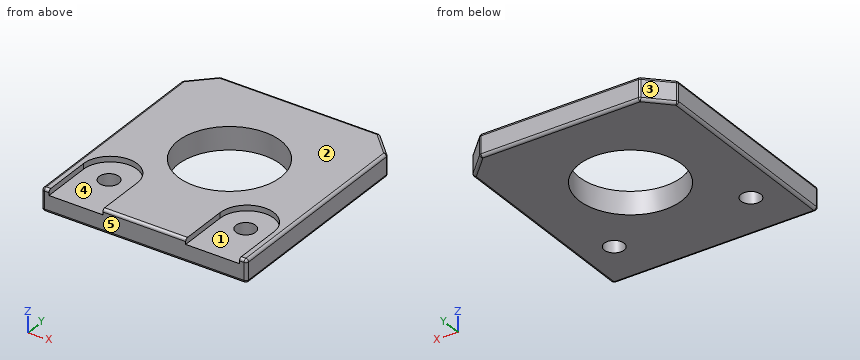
```python
from build123d import *

# Parameters (mm, degrees)
SKETCH2_W            = 57.15
SKETCH2_H            = 6.35
BOSS_EXTRUDE1_DEPTH  = 63.5
SKETCH3_R            = 14.2875
CUT_EXTRUDE1_DEPTH   = 70.922121857
CHAMFER1_SIZE        = 6.35
M5_CLEARANCE_HOLE1_D = 5.5
FILLET1_R            = 0.762
CUT_EXTRUDE4_DEPTH   = 1.524


with BuildPart() as part:
    # Sketch2 → Boss-Extrude1 (new body)
    with BuildSketch(Plane(origin=(0, 0, 0), x_dir=(1, 0, 0), z_dir=(0, 1, 0))):
        Rectangle(SKETCH2_W, SKETCH2_H)
    extrude(amount=-BOSS_EXTRUDE1_DEPTH)

    # Sketch3 → Cut-Extrude1 (cut, through all)
    with BuildSketch(Plane.XY.offset(3.175)):
        with Locations((0, -28.8150046)):
            Circle(SKETCH3_R)
    extrude(amount=-CUT_EXTRUDE1_DEPTH, mode=Mode.SUBTRACT)

    # Chamfer1
    chamfer1_edges = [part.edges().sort_by_distance(p)[0] for p in [
        (28.575, 0, 0),
        (-28.575, 0, 0),
    ]]
    chamfer(chamfer1_edges, length=CHAMFER1_SIZE)

    # M5 Clearance Hole1 (through all)
    with Locations(Plane.XY.offset(3.175)):
        with Locations((-19.05, -50.000003124), (19.05, -50.000003124)):
            Hole(M5_CLEARANCE_HOLE1_D / 2)

    # Fillet1
    fillet1_edges = [part.edges().sort_by_distance(p)[0] for p in [
        (28.575, -63.5, 0),
        (0, -63.5, -3.175),
        (0, 0, 3.175),
        (0, 0, -3.175),
        (22.225, 0, 0),
        (-22.225, 0, 0),
        (25.4, -3.175, 3.175),
        (-25.4, -3.175, 3.175),
        (-28.575, -6.35, 0),
        (25.4, -3.175, -3.175),
        (-25.4, -3.175, -3.175),
        (28.575, -6.35, 0),
        (-28.575, -63.5, 0),
        (-28.575, -34.925, -3.175),
        (28.575, -34.925, -3.175),
        (28.575, -34.925, 3.175),
        (-28.575, -34.925, 3.175),
        (0, -63.5, 3.175),
    ]]
    fillet(fillet1_edges, radius=FILLET1_R)

    # Sketch8 → Cut-Extrude4 (cut)
    with BuildSketch(Plane.XY.offset(3.175)):
        with BuildLine():
            Line((11.55, -63.5), (11.55, -49.5))
            ThreePointArc((11.55, -49.5), (19.05, -42), (26.55, -49.5))
            Line((26.55, -49.5), (26.55, -63.5))
            Line((26.55, -63.5), (11.55, -63.5))
        make_face()
    cut_extrude4 = extrude(amount=-CUT_EXTRUDE4_DEPTH, mode=Mode.SUBTRACT)

    # Mirror1: Cut-Extrude4 across plane
    add(cut_extrude4.mirror(Plane(origin=(0, 0, 0), x_dir=(0, 0, 1), z_dir=(1, 0, 0))), mode=Mode.SUBTRACT)


solid = part.part
```
Here's how the part is built. I have some questions about the finished solid (model axes, mm). Face numbers are marked on the shaded views. A direction names the side the tool comes from. Coordinates: 2 decimals unless noted, no trailing zeros. Loops run counter-clockwise (first coordinate to the right, second up) from the corner with the lowest first, then second, coordinate; pieces in that order, holes last. Notation, with made-up numbers: (53, 77) -> (89, 77) arc R17 cw to (89, 90) -> close; hole circle Ø1 at (88, 85.25). An arc over 180 degrees is marked (long way). Return JSON: item names as keys, results as strings.
1) Will these pins go through, and if not, where does the flat tip stop? pin 1 (2 mm diameter, centred on y = -39, z = 2.5, fed in from -X) (3 decimals); pin 2 (4.5 mm diameter, centred on x = 19.05, y = -50, fed in from +Z); pin 3 (7.5 mm diameter, centred on x = -18, y = -56, fed in from +Z).
Results below:
{"pin 1": "x = -28.575", "pin 2": "through", "pin 3": "z = 1.65"}
2) Thinking about a two-plate mould opening in X: for the marked faces 1, 2 and 3, which applies, +X half, -X half, draft (parallel to the pull), parting line (faces both ways), or undercut?
Results below:
{"face 1": "undercut", "face 2": "draft", "face 3": "-X half"}
3) If we section it at A-A, the plane x = 0: Write out the boundary of the cut face in (y, z) (1 decimal), then the cut area to 3 significant figures.
Results below:
{"outline": "(-63.5, -2.4) arc R0.8 ccw to (-62.7, -3.2) -> (-43.1, -3.2) -> (-43.1, 3.2) -> (-62.7, 3.2) arc R0.8 ccw to (-63.5, 2.4) -> close; (-14.5, -3.2) -> (-0.8, -3.2) arc R0.8 ccw to (0, -2.4) -> (0, 2.4) arc R0.8 ccw to (-0.8, 3.2) -> (-14.5, 3.2) -> close", "area": "221 mm²"}
4) If we section it at B-B, the plane y = -39: Write out the boundary of the cut face in (x, z) (3 decimals).
Results below:
{"outline": "(-28.575, -2.413) arc R0.762 ccw to (-27.813, -3.175) -> (-10.02, -3.175) -> (-10.02, 3.175) -> (-27.813, 3.175) arc R0.762 ccw to (-28.575, 2.413) -> close; (10.02, -3.175) -> (27.813, -3.175) arc R0.762 ccw to (28.575, -2.413) -> (28.575, 2.413) arc R0.762 ccw to (27.813, 3.175) -> (10.02, 3.175) -> close"}
5) If we section it at D-D, the plane y = -58.5: Write out the boundary of the cut face in (x, z) (3 decimals), then the cut area to 3 significant figures.
Results below:
{"outline": "(-28.575, -2.413) arc R0.762 ccw to (-27.813, -3.175) -> (27.813, -3.175) arc R0.762 ccw to (28.575, -2.413) -> (28.575, 2.413) arc R0.762 ccw to (27.813, 3.175) -> (26.55, 3.175) -> (26.55, 1.651) -> (11.55, 1.651) -> (11.55, 3.175) -> (-11.55, 3.175) -> (-11.55, 1.651) -> (-26.55, 1.651) -> (-26.55, 3.175) -> (-27.813, 3.175) arc R0.762 ccw to (-28.575, 2.413) -> close", "area": "317 mm²"}
6) For the marked faces 4 and 5, which set-ups out of +Z, -Z, +X, -X, +Y, -Y let a thin tool reach every point of the face, with its end or its side?
Results below:
{"face 4": "+Z, -Y", "face 5": "+Z, -Z, +X, -X, -Y"}
7) I need wall thicknesses on line 1 (X direction, y = -60.5, z = 1.75) (3 decimals); line 2 (Y direction, x = 0, z = 1.5); line 3 (Y direction, x = -19.05, z = -2.1). Which ranges of each line are inside material? Lowest first, please. Write a range as from..to.
Results below:
{"line 1": "-28.575..-26.55, -11.55..11.55, 26.55..28.575", "line 2": "-63.5..-43.1, -14.53..0", "line 3": "-63.5..-52.75, -47.25..0"}
8) If we section it at C-C, the plane z = 0.5: Count the separate pieces of the cut face and the enclosed holes in it, then the cut area to 3 significant figures.
Results below:
{"separate pieces": "1", "enclosed holes": "3", "area": "2,900 mm²"}
